Source: CAD feature listing. Evaluate the final solid. Frame: model axes, mm. Round coordinates to 2 decimals unless told otherwise and drop trailing zeros. Write each loop counter-clockwise with the first axis right and the second up, starting at its lowest first coordinate (ties: lowest second). Pieces come first, ordered by that corner, then holes.
```python
from build123d import *

# Parameters (mm, degrees)
SKETCH1_W            = 42
SKETCH1_H            = 42
BOSS_EXTRUDE1_DEPTH  = 6
M3_CLEARANCE_HOLE1_D = 3.2
SKETCH6_R            = 11
CUT_EXTRUDE3_DEPTH   = 7
FILLET1_R            = 5


with BuildPart() as part:
    # Sketch1 → Boss-Extrude1 (new body)
    with BuildSketch(Plane(origin=(0, 0, 0), x_dir=(1, 0, 0), z_dir=(0, 1, 0))):
        Rectangle(SKETCH1_W, SKETCH1_H)
    extrude(amount=BOSS_EXTRUDE1_DEPTH)

    # M3 Clearance Hole1 (through all)
    with Locations(Plane(origin=(0, 0, 0), x_dir=(0, 0, -1), z_dir=(0, -1, 0))):
        with Locations((15.5, -15.5), (-15.5, -15.5), (-15.5, 15.5), (15.5, 15.5)):
            Hole(M3_CLEARANCE_HOLE1_D / 2)

    # Sketch6 → Cut-Extrude3 (cut, through all)
    with BuildSketch(Plane(origin=(0, 0, 0), x_dir=(0, 0, 1), z_dir=(0, -1, 0))):
        Circle(SKETCH6_R)
    extrude(amount=-CUT_EXTRUDE3_DEPTH, mode=Mode.SUBTRACT)

    # Fillet1
    fillet1_edges = [part.edges().sort_by_distance(p)[0] for p in [
        (21, 3, 21),
        (-21, 3, 21),
        (-21, 3, -21),
        (21, 3, -21),
    ]]
    fillet(fillet1_edges, radius=FILLET1_R)


solid = part.part
```
Q1. Line query: line 1 (X direction, y = 1.5, z = -15.5); line 2 (Z direction, x = -15, y = 5); line 3 (X direction, y = 4.8, z = 0). Output: solid intervals per line, ascending.
Q2. Mould query, pull axis Z, two halves, no side actions, for faces 1 (the face through (-14.42, 3.04, -16.68)), 2 (the face through (-15.43, 3.04, 13.9)), 3 (the face through (0, 3, 21)), 4 (the face through (-10, 6, -10)). Classes: pulls with the +Z half, pulls with the -Z half, needs draft (parallel to the pull), parting line crosses it, or undercut.
Q3. Section query B-B, the plane z = -15.5. Output: boundary loops of the cut face in (x, y).
Q4. Section query D-D, the plane y = 2.25. Output: boundary loops of the cut face in (x, z), and give its area (3 significant figures).
Q5. Section query C-C, the plane x = 15.5. Output: boundary loops of the cut face in (y, z).
Q6. Section query A-A, the plane x = 0. Output: boundary loops of the cut face in (y, z), and give its area (3 significant figures).
Q7. Pin query (flat end, axial travel): P1, Ø3, axis at x = 15.5, z = 15.5, coming from the -Y side. Return the tip coordinate at first contact, or that it passes through.
Filled in:
1. line 1: x = -21 to -17.1, -13.9 to 13.9, 17.1 to 21
1. line 2: z = -21 to -17.02, -13.98 to 13.98, 17.02 to 21
1. line 3: x = -21 to -11, 11 to 21
2. face 1: undercut
2. face 2: undercut
2. face 3: pulls with the +Z half
2. face 4: needs draft
3. outline: (-21, 0) - (-17.1, 0) - (-17.1, 6) - (-21, 6) - close; (-13.9, 0) - (13.9, 0) - (13.9, 6) - (-13.9, 6) - close; (17.1, 0) - (21, 0) - (21, 6) - (17.1, 6) - close
4. outline: (-21, -16) arc R5 ccw to (-16, -21) - (16, -21) arc R5 ccw to (21, -16) - (21, 16) arc R5 ccw to (16, 21) - (-16, 21) arc R5 ccw to (-21, 16) - close; hole circle Ø3.2 at (-15.5, -15.5); hole circle Ø3.2 at (-15.5, 15.5); hole circle Ø22 at (0, 0); hole circle Ø3.2 at (15.5, -15.5); hole circle Ø3.2 at (15.5, 15.5)
4. area: 1,330 mm2
5. outline: (0, -21) - (6, -21) - (6, -17.1) - (0, -17.1) - close; (0, -13.9) - (6, -13.9) - (6, 13.9) - (0, 13.9) - close; (0, 17.1) - (6, 17.1) - (6, 21) - (0, 21) - close
6. outline: (0, -21) - (6, -21) - (6, -11) - (0, -11) - close; (0, 11) - (6, 11) - (6, 21) - (0, 21) - close
6. area: 120 mm2
7. P1: passes through
